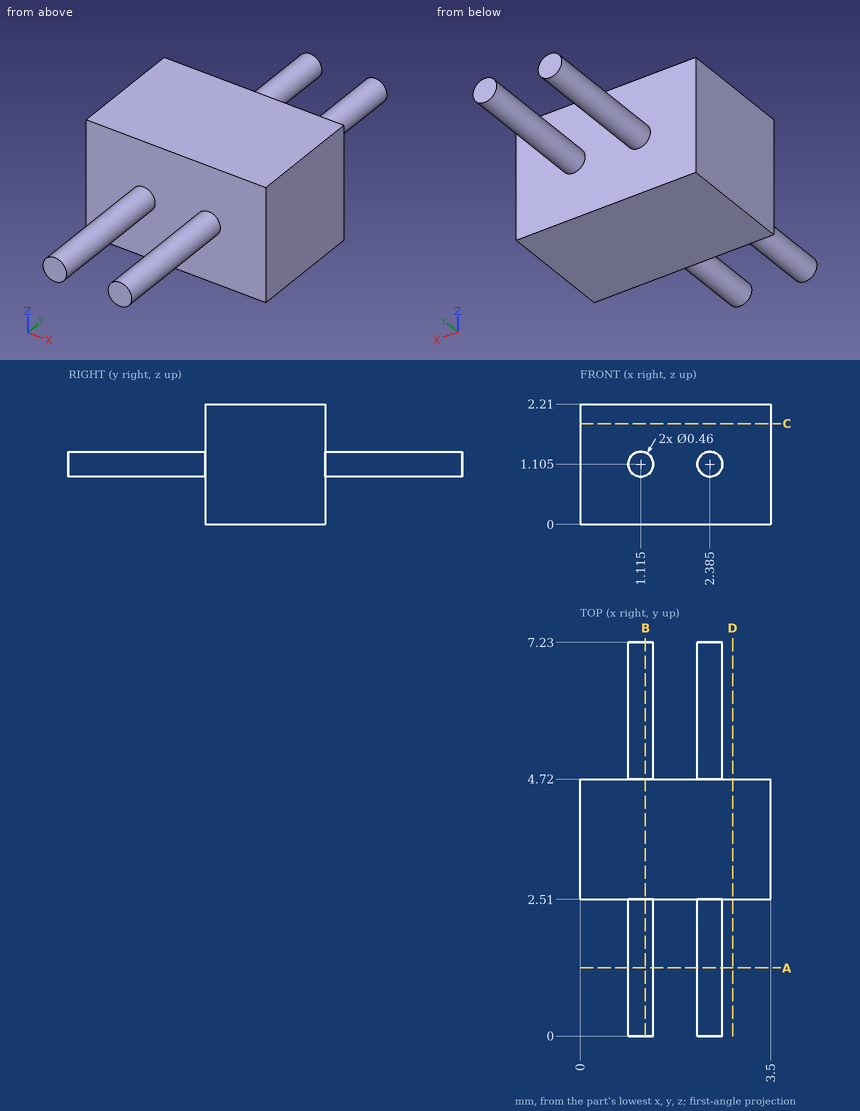
Input: dimensioned drawing with shaded views. Units: mm. Origin: part minimum x, y, z. Give positions to 0.01 mm unless a question says otherwise; leave off trailing zeros. Write each loop counter-clockwise with the first axis right and the second up, starting at its lowest first coordinate (ties: lowest second). Pieces come first, ordered by that corner, then holes. Notation, with made-up numbers: (-40, 53) -> (-14, 53) arc R21 cw to (-14, 76) -> close; hole circle Ø3 at (-8, 81.5). An arc over 180 degrees is marked (long way). Answer as a JSON object with one key per item and string values.
1. Cut plane C-C on z = 1.85. Output: boundary loops of the cut face in (x, y), and give its area (4 significant figures).
Ans:
{"outline": "(0, 2.51) -> (3.5, 2.51) -> (3.5, 4.72) -> (0, 4.72) -> close", "area": "7.735 mm^2"}
2. Contact query for flat-ended pins moving along their axis: pin 1 (2 mm diameter, centred on x = 0.5, y = 1, fed in from +Z) (3 decimals); pin 2 (1 mm diameter, centred on x = 2.5, y = 6, fed in from -Z) (3 decimals). Output: stop coordinate, or through.
Ans:
{"pin 1": "stops at z = 1.335", "pin 2": "stops at z = 0.875"}
3. Cut plane D-D on x = 2.8. Output: boundary loops of the cut face in (y, z), and give its area (3 significant figures).
Ans:
{"outline": "(2.51, 0) -> (4.72, 0) -> (4.72, 2.21) -> (2.51, 2.21) -> close", "area": "4.88 mm^2"}
4. Cut plane A-A on y = 1.25. Output: boundary loops of the cut face in (x, z) (3 decimals).
Ans:
{"outline": "circle Ø0.46 at (1.115, 1.105); circle Ø0.46 at (2.385, 1.105)"}
5. Ray query, probe 1 along Y at (x, z) = (2.6, 0.2); probe 2 along X at (y, z) = (4.75, 1.2); probe 3 along Z at (x, y) = (0.95, 6.5). Return the intervals inside material, ascending. Write a range as from..to.
Ans:
{"probe 1": "y = 2.51..4.72", "probe 2": "x = 0.91..1.32, 2.18..2.59", "probe 3": "z = 0.94..1.27"}
6. Cut plane B-B on x = 1.2. Output: boundary loops of the cut face in (y, z).
Ans:
{"outline": "(0, 0.89) -> (2.51, 0.89) -> (2.51, 0) -> (4.72, 0) -> (4.72, 0.89) -> (7.23, 0.89) -> (7.23, 1.32) -> (4.72, 1.32) -> (4.72, 2.21) -> (2.51, 2.21) -> (2.51, 1.32) -> (0, 1.32) -> close"}
